from build123d import *

# Parameters (mm, degrees)
F2_R     = 8.89
F3_DEPTH = 37.8751575137
F4_R     = 1.905
F5_DEPTH = 6.35


with BuildPart() as f1:
    # F0 (on Front) → F1 (revolve)
    with BuildSketch(Plane.XZ):
        with BuildLine():
            ThreePointArc((-0.1857913862, -31.5262409051), (-22.2928058356, -22.2928058356), (-31.5262409051, -0.1857913862))
            Line((-31.5262409051, -0.1857913862), (-37.8761306398, -0.2232127463))
            ThreePointArc((-37.8761306398, -0.2232127463), (-26.7829338961, -26.7829338961), (-0.2232127463, -37.8761306398))
            Line((-0.2232127463, -37.8761306398), (-0.1857913862, -31.5262409051))
        make_face()
    revolve(axis=Axis((-0.2045020662, 0, -34.7011857724), (-0.0058931276, 0, -0.9999826354)))

    # F2 (on Front) → F3 (cut, through all)
    with BuildSketch(Plane.XZ):
        Circle(F2_R)
    extrude(amount=-F3_DEPTH, mode=Mode.SUBTRACT)

    # F4 (on Right) → F5 (join, symmetric)
    with BuildSketch(Plane.YZ):
        with BuildLine():
            Line((-37.3891351909, -0.3715698676), (-31.5245985714, -0.3715698676))
            Line((-31.5245985714, -0.3715698676), (-29.2478017509, -0.3715698676))
            Line((-29.2478017509, -0.3715698676), (-31.0778754838, 3.9011891729))
            ThreePointArc((-31.0778754838, 3.9011891729), (-34.3635014884, 6.610138796), (-37.3891351909, 3.613592951))
            Line((-37.3891351909, 3.613592951), (-37.3891351909, 3.2632673138))
            Line((-37.3891351909, 3.2632673138), (-37.3891351909, -0.3715698676))
        make_face()
        with Locations((-34.2189706862, 3.4384301324)):
            Circle(F4_R, mode=Mode.SUBTRACT)
    extrude(amount=F5_DEPTH, both=True)


solid = f1.part
Verification items for the finished model (mm, model axes). Coordinates: 2 decimals unless noted, no trailing zeros. Write each loop counter-clockwise with the first axis right and the second up, starting at its lowest first coordinate (ties: lowest second). Pieces come first, ordered by that corner, then holes. Notation, with made-up numbers: M 64,81.5 L 96,81.5 A23 ccw 96,89.5 Z; hole C 51.5,74 d4. An arc over 180 degrees is marked long. Use a Markdown table: item, result.
Q1. Sectioned sample at B-B, the plane z = -33.5. Record the boundary of the cut face in (x, y).
Reply:
| item | result |
|---|---|
| outline | C 0,0 d35.35 |
Q2. Draft check along X on faces 1 (the face through (6.35, -32, 2)), 2 (the face through (0, -37.389, 2)), 3 (the face through (-0.243, 33.487, -8.887)). Enter one of: +X half, -X half, draft (parallel to the pull), parting line (faces both ways), or undercut.
Reply:
| item | result |
|---|---|
| face 1 | +X half |
| face 2 | draft |
| face 3 | undercut |
Q3. Sectioned sample at A-A, the plane z = -10. Record the boundary of the cut face in (x, y).
Reply:
| item | result |
|---|---|
| outline | C 0,0 d73.07; hole C 0,0 d59.8 |
Q4. Thickness scan on line 1 (X direction, y = 21, z = -1); line 2 (X direction, y = -11, z = -7); line 3 (Y direction, x = 5, z = -28). Record the ranges inside material, lowest first.
Reply:
| item | result |
|---|---|
| line 1 | x = -31.51 to -23.49, 23.49 to 31.51 |
| line 2 | x = -35.56 to -28.7, 28.7 to 35.56 |
| line 3 | y = -25.01 to -13.6, 13.6 to 25.01 |
Q5. Go/stop test with flat-tipped pins: P1, Ø3, axis at x = 17, z = -30, coming from the +Y side; P2, Ø6, axis at x = 14.5, y = 12.5, coming from the +Z side; P3, Ø8, axis at x = -8, y = 22.5, coming from the -Z side. Record where each tip stops, or that it passes through.
Reply:
| item | result |
|---|---|
| P1 | stops at y = 18.62 |
| P2 | stops at z = -22.44 |
| P3 | stops at z = -32.24 |
